```python
from build123d import *

# Parameters (mm, degrees)
F0_R     = 12.7
F1_DEPTH = 24.384
F2_R     = 1.9685
F3_DEPTH = 30.734
F4_R     = 1.905
F5_DEPTH = 6.35


with BuildPart() as f1:
    # F0 (on Front) → F1 (new body)
    with BuildSketch(Plane.XZ):
        Circle(F0_R)
    extrude(amount=F1_DEPTH)

    # F2 (on Front) → F3 (join)
    with BuildSketch(Plane.XZ):
        Circle(F2_R)
    extrude(amount=F3_DEPTH)

    # F4 (on Front) → F5 (join)
    with BuildSketch(Plane.XZ):
        Circle(F4_R)
    extrude(amount=-F5_DEPTH)


solid = f1.part
```
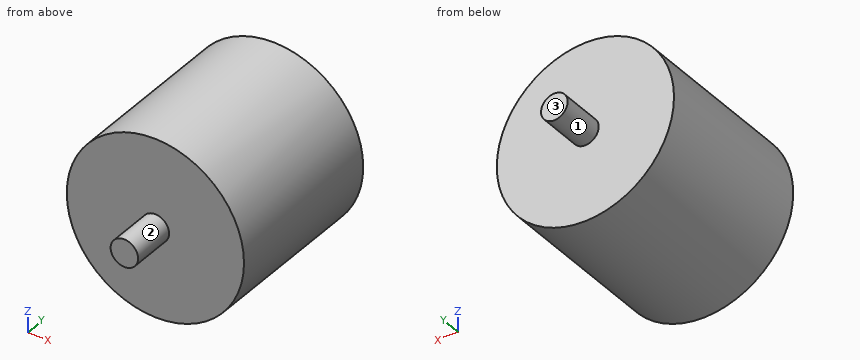
Check sheet for the modelled part. Datum: model origin and axes. Units: mm. Face numbers are marked on the shaded views. A direction names the side the tool comes from. Coordinates: 2 decimals unless noted, no trailing zeros. Order: outer loops, then holes, each group sorted by start corner. A loop starts at its lowest first (then second) coordinate and runs counter-clockwise, first axis right, second up. Notation, with made-up numbers: (-16, 1.5) -> (39, 1.5) arc R26 cw to (39, 36.5) -> close; hole circle Ø8 at (-15.5, 47.5). An arc over 180 degrees is marked (long way). Write each question's results on one line, items separated by ' | '. Start each with the question number.
1) Section check D-D (y = -26.5). Enter the section's corners in (x, z).
2) Material ranges on line 1 along Y through (x, z) = (11.25, -5.5); line 2 along Z through (x, y) = (0.5, -24); line 3 along X through (y, z) = (-22, -3), recorded low to high.
3) Set-up check for the marked faces 1, 2 and 3: record each of +Z, -Z, +X, -X, +Y, -Y from which the full face is reachable in a straight line by a thin tool's end or side.
4) Depth check by flat-ended pin: pin 1 (6 mm diameter, centred on x = 2.5, z = 6.5, fed in from -Y); pin 2 (2 mm diameter, centred on x = 2, y = -8, fed in from -Z); pin 3 (10 mm diameter, centred on y = -15, z = 5.5, fed in from -X). Enter the tip coordinate at first touch or a pass-through.
5) Section check C-C (y = -16). Enter the section's corners in (x, z), and give its area (3 significant figures).
Checked values:
1) outline: circle Ø3.94 at (0, 0)
2) line 1: -24.38 to 0 | line 2: -12.69 to 12.69 | line 3: -12.34 to 12.34
3) face 1: +Y | face 2: -Y | face 3: +Z, -Z, +X, -X, +Y
4) pin 1: y = -24.38 | pin 2: z = -12.66 | pin 3: x = -12.69
5) outline: circle Ø25.4 at (0, 0) | area: 507 mm²
